Autodesk Inventor part; units mm, degrees
ref_plane "YZ Plane" through (0, 0, 0) normal (1, 0, 0) x (0, 1, 0)
ref_plane "XZ Plane" through (0, 0, 0) normal (0, 1, 0) x (-1, 0, 0)
ref_plane "XY Plane" through (0, 0, 0) normal (0, 0, 1) x (1, 0, 0)
sketch "Sketch1" plane through (0, 0, 0) normal (0, 0, 1) x (1, 0, 0)
  line L0 (-58.4998, -9.3705) -> (144.5002, -9.3705)
  line L1 (144.5002, -9.3705) -> (144.5002, -119.3705)
  line L2 (144.5002, -119.3705) -> (-58.4998, -119.3705)
  line L3 (-58.4998, -119.3705) -> (-58.4998, -9.3705)
  line L4 (-58.4998, -9.3705) -> (-38.4998, -9.3705)
  line L5 (-38.4998, -9.3705) -> (-38.4998, -21.3705)
  line L6 (-38.4998, -21.3705) -> (-58.4998, -21.3705)
  line L7 (-58.4998, -21.3705) -> (-58.4998, -9.3705)
  line L8 (144.5002, -9.3705) -> (124.5002, -9.3705)
  line L9 (124.5002, -9.3705) -> (124.5002, -21.3705)
  line L10 (124.5002, -21.3705) -> (144.5002, -21.3705)
  line L11 (144.5002, -21.3705) -> (144.5002, -9.3705)
  circle A0 centre (-56.009, -27.3705) radius 2
  circle A1 centre (142.0094, -27.3705) radius 2
  circle A2 centre (43.0002, -17.3705) radius 2
  circle A3 centre (-56.009, -111.8705) radius 2
  circle A4 centre (42.0002, -111.8705) radius 2
  circle A5 centre (142.0094, -113.8705) radius 2
  point P0 (0, 0)
  dimension "d0" = 203
  dimension "d1" = 110
  dimension "d2" = 20
  dimension "d3" = 12
  dimension "d4" = 20
  dimension "d5" = 12
  dimension "d6" = 4
  dimension "d7" = 4
  dimension "d8" = 198.0184
  dimension "d9" = 2.4908
  dimension "d10" = 18
  dimension "d11" = 4
  dimension "d12" = 10
  dimension "d13" = 99.0092
  dimension "d14" = 4
  dimension "d15" = 84.5
  dimension "d16" = 4
  dimension "d17" = 4
  dimension "d18" = 0
extrude "Extrusion1" add sketch "Sketch1" along normal blind 2 contours L0 L9 L10 L1 L2 L3 L6 L5
sketch "Sketch3" plane through (0, 0, 0) normal (0, 0, -1) x (-1, 0, 0)
  circle A0 centre (56.009, -111.8705) radius 2
  circle A1 centre (-42.0002, -111.8705) radius 2
  circle A2 centre (-142.0094, -113.8705) radius 2
  circle A3 centre (-142.0094, -27.3705) radius 2
  circle A4 centre (-43.0002, -17.3705) radius 2
  circle A5 centre (56.009, -27.3705) radius 2
  circle A6 centre (56.009, -111.8705) radius 6
  circle A7 centre (-42.0002, -111.8705) radius 6
  circle A8 centre (-142.0094, -113.8705) radius 2
  circle A9 centre (-142.0094, -113.8705) radius 6
  circle A10 centre (-43.0002, -17.3705) radius 6
  circle A11 centre (-142.0094, -27.3705) radius 6
  circle A12 centre (56.009, -27.3705) radius 6
  circle A13 centre (56.009, -111.8705) radius 4
  circle A14 centre (-42.0002, -111.8705) radius 4
  circle A15 centre (56.009, -27.3705) radius 4
  circle A16 centre (-43.0002, -17.3705) radius 4
  circle A17 centre (-142.0094, -27.3705) radius 4
  circle A18 centre (-142.0094, -113.8705) radius 4
  point P0 (0, 0)
  dimension "d45" = 12
  dimension "d46" = 12
  dimension "d47" = 12
  dimension "d48" = 12
  dimension "d49" = 12
  dimension "d50" = 12
  dimension "d51" = 8
  dimension "d52" = 8
  dimension "d53" = 8
  dimension "d54" = 8
  dimension "d55" = 8
  dimension "d56" = 8
extrude "Extrusion3" add sketch "Sketch3" along normal blind 3 contours A6 | A7 | A9 | A10 | A11 | A12
sketch "Sketch4" plane through (0, 0, 2) normal (0, 0, 1) x (1, 0, 0)
  line L0 (124.5002, -9.3705) -> (-38.4998, -9.3705)
  line L1 (-38.4998, -9.3705) -> (-38.4998, -21.3705)
  line L2 (-38.4998, -21.3705) -> (-58.4998, -21.3705)
  line L3 (-58.4998, -21.3705) -> (-58.4998, -119.3705)
  line L4 (-58.4998, -119.3705) -> (144.5002, -119.3705)
  line L5 (144.5002, -119.3705) -> (144.5002, -21.3705)
  line L6 (144.5002, -21.3705) -> (124.5002, -21.3705)
  line L7 (124.5002, -21.3705) -> (124.5002, -9.3705)
  line L8 (-77.131, 13.4165) -> (211.8208, 13.4165)
  line L9 (211.8208, 13.4165) -> (211.8208, -174.2275)
  line L10 (211.8208, -174.2275) -> (-77.131, -174.2275)
  line L11 (-77.131, -174.2275) -> (-77.131, 13.4165)
  point P0 (0, 0)
extrude "Extrusion4" cut sketch "Sketch4" against normal through all
sketch "Sketch6" plane through (0, 0, 2) normal (0, 0, 1) x (1, 0, 0)
  circle A0 centre (-38.4998, -99.9669) radius 1.5
  circle A1 centre (-38.4998, -41.9669) radius 1.5
  line L0 (-58.4998, -21.3705) -> (-58.4998, -119.3705)
  circle A2 centre (10.5002, -99.9669) radius 1.5
  circle A3 centre (10.5002, -41.9669) radius 1.5
  point P0 (0, 0)
  dimension "d73" = 3
  dimension "d74" = 3
  dimension "d75" = 20
  dimension "d76" = 20
  dimension "d77" = 58
  dimension "d78" = 3
  dimension "d79" = 49
  dimension "d80" = 3
extrude "Extrusion6" cut sketch "Sketch6" against normal blind 10
sketch "Sketch8" plane through (0, 0, 2) normal (0, 0, 1) x (1, 0, 0)
  line L0 (-58.4998, -119.3705) -> (144.5002, -119.3705)
  line L1 (144.5002, -119.3705) -> (-58.4998, -119.3705)
  line L2 (-58.4998, -119.3705) -> (-58.4998, -149.3705)
  line L3 (-58.4998, -149.3705) -> (144.5002, -149.3705)
  line L4 (144.5002, -149.3705) -> (144.5002, -119.3705)
  point P0 (0, 0)
  dimension "d86" = 30
extrude "Extrusion7" add sketch "Sketch8" against normal blind 2
sketch "Sketch9" plane through (0, 0, 2) normal (0, 0, 1) x (1, 0, 0)
  circle A0 centre (104.5002, -24.3705) radius 2.25
  circle A1 centre (104.5002, -139.0705) radius 2.25
  line L0 (124.5002, -9.3705) -> (-38.4998, -9.3705)
  line L1 (144.5002, -149.3705) -> (144.5002, -21.3705)
  point P0 (0, 0)
  dimension "d89" = 4.5
  dimension "d90" = 4.5
  dimension "d91" = 15
  dimension "d92" = 114.7
  dimension "d93" = 40
  dimension "d94" = 40
extrude "Extrusion8" cut sketch "Sketch9" against normal blind 2
equation "\"d13\" = 0.5 * d8"
properties part number "PiAndBusBarPlate"
Verification items for the finished model (mm, model axes). A direction names the side the tool comes from. Round coordinates to 2 decimals unless told otherwise and drop trailing zeros. Order: outer loops, then holes, each group sorted by start corner. A loop starts at its lowest first (then second) coordinate and runs counter-clockwise, first axis right, second up.
1. Section check A-A on z = -2.15. Record the cut outline in (x, y).
Final values:
outline: (-58.5, -117.33) arc R6 ccw (long way) to (-58.5, -106.41) - (-58.5, -108.74) arc R4 cw (long way) to (-58.5, -115) - close; (-58.5, -32.83) arc R6 ccw (long way) to (-58.5, -21.91) - (-58.5, -24.24) arc R4 cw (long way) to (-58.5, -30.5) - close; circle Ø12 at (42, -111.87); circle Ø12 at (43, -17.37); (139.61, -119.37) - (144.41, -119.37) arc R6 ccw to (144.5, -119.33) - (144.5, -117) arc R4 cw (long way) to (144.5, -110.74) - (144.5, -108.41) arc R6 ccw (long way) to start; (144.5, -32.83) - (144.5, -30.5) arc R4 cw (long way) to (144.5, -24.24) - (144.5, -21.91) arc R6 ccw (long way) to start; hole circle Ø8 at (42, -111.87); hole circle Ø8 at (43, -17.37)
2. Section check C-C on x = 51.5. Record the cut outline in (y, z), then the cut area to 3 significant figures.
Final values:
outline: (-149.37, 0) - (-9.37, 0) - (-9.37, 2) - (-149.37, 2) - close
area: 280 mm2
3. Thickness scan on L1, parallel to Y at x = -38, z = 0.45; L2, parallel to Z at x = 5, y = -72; L3, parallel to Y at x = 134.5, z = 0.55. Record the ranges inside material, lowest first.
Final values:
L1: y = -149.37 to -101.38, -98.55 to -43.38, -40.55 to -9.37
L2: z = 0 to 2
L3: y = -149.37 to -21.37
4. Release check for a two-part mould opening along X. For faces 3 (the flat face through (137, -114, -3)), 4 (the flat face through (-58.5, -84, 1)), 5 (the cylindrical face through (40.85, -20.743, -1.479)) record: +X half, -X half, draft (parallel to the pull), parting line (faces both ways), or undercut.
Final values:
face 3: draft
face 4: -X half
face 5: undercut
5. Go/stop test with flat-tipped pins: P1, Ø0.6, axis at y = -13.5, z = 0.5, coming from the +X side; P2, Ø4.5, axis at x = -56.01, y = -111.87, coming from the -Z side; P3, Ø0.6, axis at x = 132.5, z = 1.5, coming from the +Y side. Record where each tip stops, or that it passes through.
Final values:
P1: stops at x = 124.5
P2: stops at z = 0
P3: stops at y = -21.37
6. Section check B-B on y = -52.5. Record the cut outline in (x, z), then the cut area to 3 significant figures.
Final values:
outline: (-58.5, 0) - (144.5, 0) - (144.5, 2) - (-58.5, 2) - close
area: 406 mm2
7. Access from +Z, -Z, +X, -X, +Y, -Y to the whole of each face (thin tool, end or side, straight path). Record for faces 1 (the cylindrical face through (-52.01, -27.5, -1.48)), 2 (the flat face through (41, -116, -3)).
Final values:
face 1: -Z
face 2: -Z, +X, -X, +Y, -Y
